Geometry: final body of the model. Coordinates: model frame, mm. A direction names the side the tool comes from. Give positions to 0.01 mm unless a question says otherwise; leave off trailing zeros. Write each loop counter-clockwise with the first axis right and the second up, starting at its lowest first coordinate (ties: lowest second). Pieces come first, ordered by that corner, then holes.
Q1. Reachability of faces 4 (the face through (0, 0, 27)), 5 (the face through (-20, -19, -7)) from +Z, -Z, +X, -X, +Y, -Y: full face, straight path, thin tool, end or side. Return the list, or none.
Q2. Line query: L1, parallel to Y at x = -5.5, z = 0; L2, parallel to Z at x = -5, y = 0; L3, parallel to Z at x = 13, y = -12.5. Output: solid intervals per line, ascending.
Q3. Cut plane A-A on y = 0. Return the cut outline in (x, z).
Q4. Cut plane D-D on x = 14. Return the cut outline in (y, z), plus the area to 3 significant figures.
Q5. Cut plane C-C on x = 8.5. Return the cut outline in (y, z), plus the area to 3 significant figures.
Q6. Draft query along Y for faces 1 (the face through (20, -19, 7)), 2 (the face through (-0.21, 10.724, 25.865)), 3 (the face through (0.28, 19.524, -4.336)). Return one class per face: pulls with the +Y half, pulls with the -Y half, needs draft (parallel to the pull), parting line crosses it, or undercut.
Q7. Cut plane B-B on z = 0. Return the cut outline in (x, y).
Q8. Pin query (flat end, axial travel): pin 1 (9.5 mm diameter, centred on x = 0, y = -1, fed in from +Z); pin 2 (4 mm diameter, centred on x = -11.5, z = 3, fed in from +Y); pin 3 (8 mm diameter, centred on x = 9.5, y = 22, fed in from +Z). Return the tip coordinate at first contact, or that it passes through.
```python
from build123d import *

# Parameters (mm, degrees)
F0_W     = 24
F0_H     = 1
F2_R     = 5
F3_DEPTH = 6


with BuildPart() as f1:
    # F0 (on Front) → F1 (revolve)
    with BuildSketch(Plane.XZ):
        Polygon((-20, 28), (-20, 20), (0, 20), (20, 20), (20, 28), (12, 28), (12, 27), (-12, 27), (-12, 28), align=None)
        with Locations((0, 27.5)):
            Rectangle(F0_W, F0_H)
    revolve(axis=Axis((2.7690531401, 0, 0), (1, 0, 0)))

    # F2
    f2_edges = [f1.edges().sort_by_distance(p)[0] for p in [
        (20, 0, -28),
        (-20, 0, -28),
    ]]
    fillet(f2_edges, radius=F2_R)

    # F0 (on Front) → F3 (cut, symmetric)
    with BuildSketch(Plane.XZ):
        with Locations((0, 27.5)):
            Rectangle(F0_W, F0_H)
    extrude(amount=F3_DEPTH, both=True, mode=Mode.SUBTRACT)


solid = f1.part
```
Data:
1. face 4: +Z
1. face 5: +Z, -Z, -X, +Y, -Y
2. L1: y = -28 to -20, 20 to 28
2. L2: z = -28 to -20, 20 to 27
2. L3: z = -25.05 to -15.61, 15.61 to 25.05
3. outline: (-20, -23) arc R5 ccw to (-15, -28) - (15, -28) arc R5 ccw to (20, -23) - (20, -20) - (-20, -20) - close; (-20, 20) - (20, 20) - (20, 23) arc R5 ccw to (15, 28) - (12, 28) - (12, 27) - (-12, 27) - (-12, 28) - (-15, 28) arc R5 ccw to (-20, 23) - close
4. outline: circle Ø56 at (0, 0); hole circle Ø40 at (0, 0)
4. area: 1,210 mm2
5. outline: (-6, 27) - (-6, 27.35) arc R28 ccw (long way) to (6, 27.35) - (6, 27) - close; hole circle Ø40 at (0, 0)
5. area: 1,200 mm2
6. face 1: needs draft
6. face 2: parting line crosses it
6. face 3: undercut
7. outline: (-20, -23) arc R5 ccw to (-15, -28) - (15, -28) arc R5 ccw to (20, -23) - (20, -20) - (-20, -20) - close; (-20, 20) - (20, 20) - (20, 23) arc R5 ccw to (15, 28) - (-15, 28) arc R5 ccw to (-20, 23) - close
8. pin 1: stops at z = 27
8. pin 2: stops at y = 27.98
8. pin 3: stops at z = 21.45
